Source: CAD feature listing. Evaluate the final solid. Frame: model axes, mm. Face numbers are marked on the shaded views. A direction names the side the tool comes from. Round coordinates to 2 decimals unless told otherwise and drop trailing zeros. Loops run counter-clockwise (first coordinate to the right, second up) from the corner with the lowest first, then second, coordinate; pieces in that order, holes last. Notation, with made-up numbers: (11.5, -1) -> (64.5, -1) arc R20 ccw to (64.5, 19) -> close; hole circle Ø1 at (74.25, 66.25). An arc over 180 degrees is marked (long way). Return JSON: item names as keys, results as strings. Group by question number.
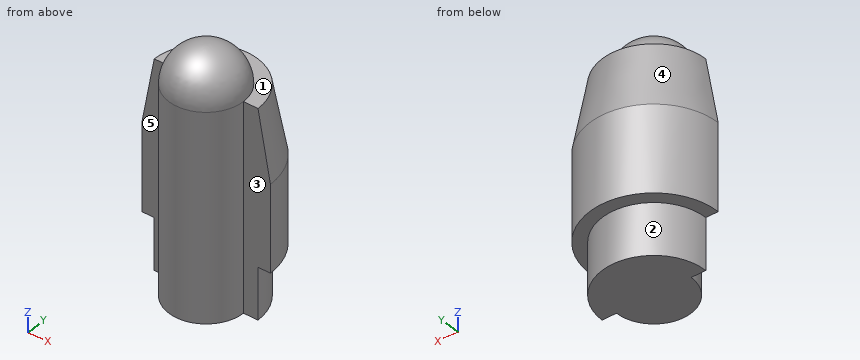
```python
from build123d import *

# Parameters (mm, degrees)
F2_ANGLE = 180


with BuildPart() as f1:
    # F0 (on Front) → F1 (revolve)
    with BuildSketch(Plane.XZ):
        with BuildLine():
            ThreePointArc((0, 10.416769), (-1.616446, 9.747216), (-2.286, 8.130769))
            Line((-2.286, 8.130769), (-2.286, -4.569231))
            Line((-2.286, -4.569231), (0, -4.569231))
            Line((0, -4.569231), (0, 10.416769))
        make_face()
    revolve(axis=Axis((0, 0, 2.689288), (0, 0, -1)))

    # F0 (on Front) → F2 (revolve)
    with BuildSketch(Plane.XZ):
        Polygon((-2.286, -4.569231), (-2.286, 8.130769), (-3.175, 8.130817), (-3.937, 3.939769), (-3.937, -1.394231), (-3.175, -1.394231), (-3.175, -4.569231), align=None)
    revolve(axis=Axis((0, 0, 2.689288), (0, 0, -1)), revolution_arc=F2_ANGLE)


solid = f1.part
```
(1) Set-up query: the marked faces 3, 4 and 5. Return all of +Z, -Z, +X, -X, +Y, -Y with unobstructed straight access to the full face (end or side cutting, diameter ignored); none if empty.
(2) Cut plane A-A (z = -1). Return loops of the section in (x, y).
(3) Mould query, pull axis X, two halves, no side actions, for the marked faces 1 and 2. Classes: released by +X, released by -X, zero draft, split by the parting line, or undercut.
(4) Cut plane B-B (z = 6.75). Return loops of the section in (x, y).
(5) Ray query, line 1 (Z direction, x = 0.75, y = 3); line 2 (Y direction, x = 2, z = -4); line 3 (X direction, y = 0.75, z = 8.75). Return the intervals inside material, ascending.
(6) Pin query (flat end, axial travel): pin 1 (0.8 mm diameter, centred on x = 3.5, z = 2.5, fed in from -Y); pin 2 (1.5 mm diameter, centred on x = -2.5, y = 1, fed in from +Z); pin 3 (4 mm diameter, centred on x = -2, z = 9, fed in from -Y). Return the tip coordinate at first contact, or that it passes through.
Answers follow:
{
 "1": {"face 3": "+Z, -Z, +X, -Y", "face 4": "+Z, +Y", "face 5": "+Z, -Z, -X, -Y"},
 "2": {"outline": "(-3.94, 0) -> (-2.29, 0) arc R2.29 ccw to (2.29, 0) -> (3.94, 0) arc R3.94 ccw to start"},
 "3": {"face 1": "zero draft", "face 2": "split by the parting line"},
 "4": {"outline": "(-3.43, 0) -> (-2.29, 0) arc R2.29 ccw to (2.29, 0) -> (3.43, 0) arc R3.43 ccw to start"},
 "5": {"line 1": "-4.57 to 8.13", "line 2": "-1.11 to 2.47", "line 3": "-2.07 to 2.07"},
 "6": {"pin 1": "y = 0", "pin 2": "z = 9.34", "pin 3": "y = -2.28"}
}
